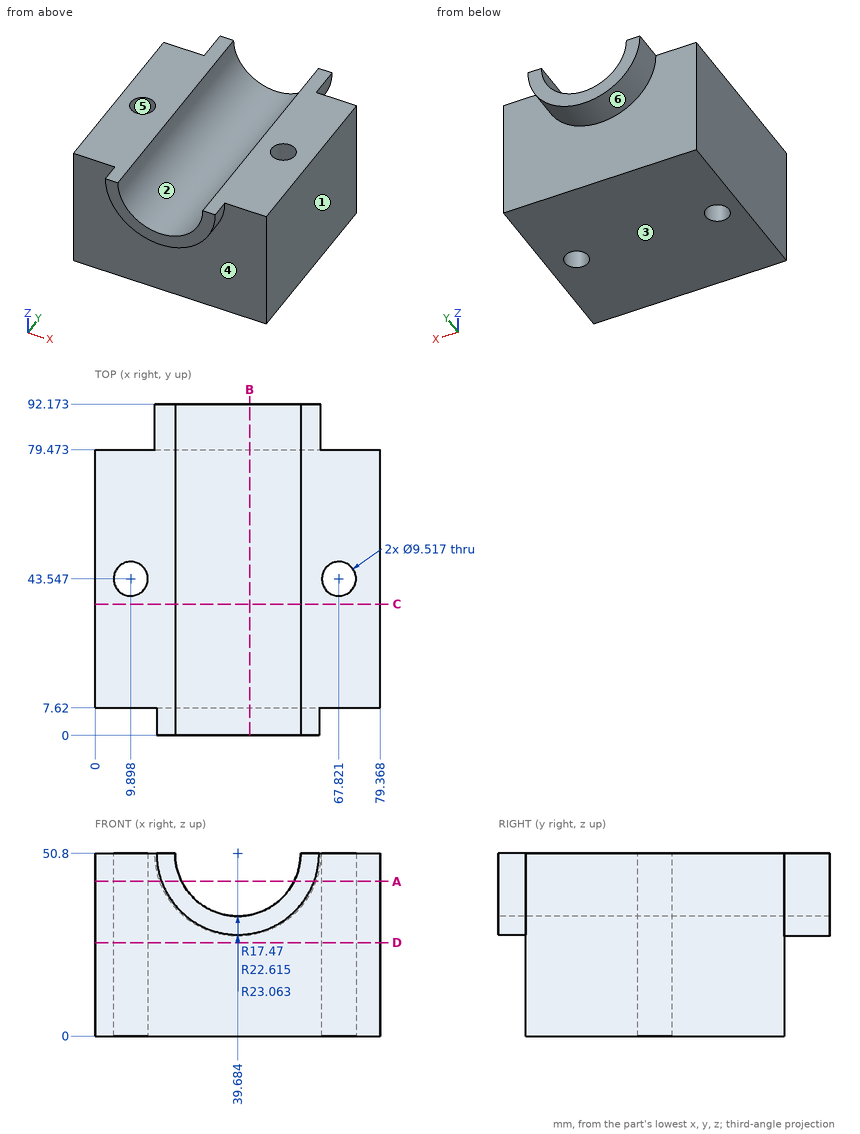
Here's the drawing with two shaded views (mm, measured from the low corner). I have some questions. A direction names the side the tool comes from. Coordinates: 2 decimals unless noted, no trailing zeros. Write each loop counter-clockwise with the first axis right and the second up, starting at its lowest first coordinate (ties: lowest second). Pieces come first, ordered by that corner, then holes. Notation, with made-up numbers: (40.5, -23) -> (95.5, -23) arc R17 cw to (95.5, 10) -> close; hole circle Ø6 at (34.5, 23). An arc over 180 degrees is marked (long way). Use a Markdown table: item, result. Add a question column.
(1) If we section it at D-D, the plane z = 26: Write out the boundary of the cut face in (x, y).
(2) For the marked faces 4, 5 and 6, which set-ups out of +Z, -Z, +X, -X, +Y, -Y let a thin tool reach every point of the face, with its end or its side?
(3) If we section it at B-B, the plane x = 43: Write out the boundary of the cut face in (y, z), and give its area (3 significant figures).
(4) If we section it at C-C, the plane y = 36.5: Write out the boundary of the cut face in (x, z) (1 decimal), and give its area (3 significant figures).
(5) We'd pull the mould along X, two halves only. Please class the marked faces 1, 2 and 3: +X half, -X half, draft (parallel to the pull), parting line (faces both ways), or undercut.
(6) If we section it at A-A, the plane z = 43: Write out the boundary of the cut face in (x, y).
(7) Please list where these lines run through material, in increasing order: line 1 (Y direction, x = 17, z = 30); line 2 (X direction, y = 41, z = 22.5); line 3 (X direction, y = 86, z = 47.5).
(8) I'm going to push flat-ended pins straight in: P1, Ø8.5, axis at x = 9.9, y = 43.55, coming from the +Z side; P2, Ø5, axis at x = 32, z = 24.5, coming from the -Y side; P3, Ø1, axis at x = 66.5, z = 7.5, coming from the +Y side; P4, Ø10, axis at x = 28.5, y = 23, coming from the +Z side (1 decimal). Where does each tip first touch, or does it pass through?
Outcome:
| question | item | result |
|---|---|---|
| 1 | outline | (0, 7.62) -> (79.37, 7.62) -> (79.37, 79.47) -> (0, 79.47) -> close; hole circle Ø9.52 at (9.9, 43.55); hole circle Ø9.52 at (67.82, 43.55) |
| 2 | face 4 | -Z, -Y |
| 2 | face 5 | +Z, -Z |
| 2 | face 6 | -Z, +Y |
| 3 | outline | (0, 28.43) -> (7.62, 28.43) -> (7.62, 0) -> (79.47, 0) -> (79.47, 27.98) -> (92.17, 27.98) -> (92.17, 33.65) -> (0, 33.65) -> close |
| 3 | area | 2,530 mm^2 |
| 4 | outline | (0, 0) -> (79.4, 0) -> (79.4, 50.8) -> (57.2, 50.8) arc R17.5 cw to (22.2, 50.8) -> (0, 50.8) -> close |
| 4 | area | 3,550 mm^2 |
| 5 | face 1 | +X half |
| 5 | face 2 | undercut |
| 5 | face 3 | draft |
| 6 | outline | (0, 7.62) -> (18.46, 7.62) -> (18.46, 0) -> (24.05, 0) -> (24.05, 92.17) -> (17.98, 92.17) -> (17.98, 79.47) -> (0, 79.47) -> close; (55.32, 0) -> (60.91, 0) -> (60.91, 7.62) -> (79.37, 7.62) -> (79.37, 79.47) -> (61.39, 79.47) -> (61.39, 92.17) -> (55.32, 92.17) -> close; hole circle Ø9.52 at (9.9, 43.55); hole circle Ø9.52 at (67.82, 43.55) |
| 7 | line 1 | y = 7.62 to 79.47 |
| 7 | line 2 | x = 0 to 5.88, 13.92 to 63.8, 71.84 to 79.37 |
| 7 | line 3 | x = 16.86 to 22.53, 56.84 to 62.51 |
| 8 | P1 | passes through |
| 8 | P2 | stops at y = 7.62 |
| 8 | P3 | stops at y = 79.47 |
| 8 | P4 | stops at z = 44.2 |
